Can you work these out from the model? Positions are in its coordinate system, mm. Face numbers are marked on the shaded views. A direction names the side the tool comes from. Coordinates: 2 decimals unless noted, no trailing zeros. Write each loop counter-clockwise with the first axis right and the second up, starting at its lowest first coordinate (ties: lowest second). Pieces come first, ordered by that corner, then holes. Notation, with made-up numbers: (32, 38.25) - (37, 38.25) arc R19 cw to (37, 63.25) - close; hole circle Ø8 at (5, 73). An arc over 180 degrees is marked (long way). Use one line per item in the form item = value. Start each with the question number.
(1) If we section it at D-D on z = 15.5: Please give me the cut outline in (x, y).
(2) Thinking about a two-plate mould opening in X: for the marked faces 4, 5 and 6, which applies, pulls with the +X half, pulls with the -X half, needs draft (parallel to the pull), parting line crosses it, or undercut?
(3) If we section it at B-B on x = 0: Please give me the cut outline in (y, z).
(4) On a 3-axis mill with a long thin cutter (end or side, diameter ignored), from which of +Z, -Z, +X, -X, +Y, -Y can I reach the whole of each face in a straight line? I mean the marked faces 1, 2 and 3. Say none if no direction works.
(5) If we section it at A-A on z = 2.5: Please give me the cut outline in (x, y).
(6) For pin 1 Ø6 at (x, z) = (19, -10) entering from +Y; pin 2 Ø12.5 at (x, y) = (3.5, -23) entering from +Z; pin 3 Ø6.5 at (y, z) = (-56.5, -4) entering from +X; pin 4 Ø10 at (x, y) = (2, -56) entering from +Z, each with a flat end and sliding along its axis, tell me the tip position at first contact or that it passes through.
(7) If I drill on probe 1 along Y at (x, z) = (0, 14.5); probe 2 along Y at (x, z) = (-0.5, 8); probe 3 along X at (y, z) = (-26, 9.5), over which ranges is the centre line in solid material (lowest first)? Write a range as from..to.
(8) If we section it at C-C on y = -20.5: Please give me the cut outline in (x, z).
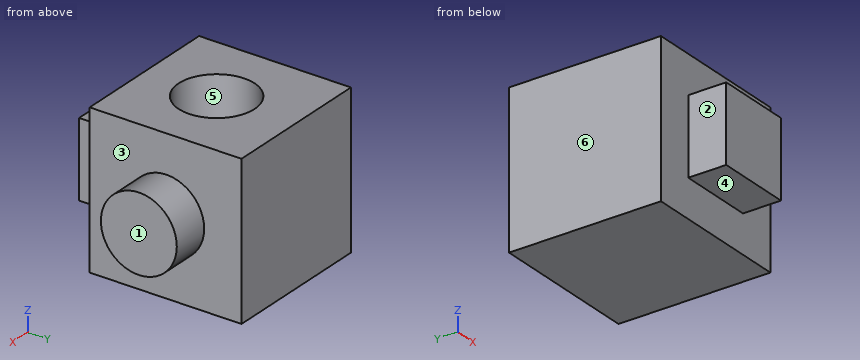
```python
from build123d import *

# Parameters (mm, degrees)
F0_W     = 50.8
F0_H     = 50.8
F1_DEPTH = 50.8
F2_W     = 25.4
F2_H     = 25.4
F3_DEPTH = 12.7
F4_R     = 12.7
F5_DEPTH = 12.7
F6_R     = 12.7
F7_DEPTH = 25.4


with BuildPart() as f1:
    # F0 (on Front) → F1 (new body)
    with BuildSketch(Plane.XZ):
        Rectangle(F0_W, F0_H)
    extrude(amount=F1_DEPTH)

    # F2 (on face) → F3 (join)
    with BuildSketch(Plane.XZ.offset(50.8)):
        Rectangle(F2_W, F2_H)
    extrude(amount=F3_DEPTH)

    # F4 (on face) → F5 (join)
    with BuildSketch(Plane.YZ.offset(25.4)):
        with Locations((-25.19346, 0)):
            Circle(F4_R)
    extrude(amount=F5_DEPTH)

    # F6 (on face) → F7 (cut)
    with BuildSketch(Plane.XY.offset(25.4)):
        with Locations((0, -26.625345)):
            Circle(F6_R)
    extrude(amount=-F7_DEPTH, mode=Mode.SUBTRACT)


solid = f1.part
```
Reported:
q1.outline = (-25.4, -50.8) - (25.4, -50.8) - (25.4, 0) - (-25.4, 0) - close; hole circle Ø25.4 at (0, -26.63)
q2.face_4 = needs draft
q2.face_5 = undercut
q2.face_6 = pulls with the -X half
q3.outline = (-63.5, -12.7) - (-50.8, -12.7) - (-50.8, -25.4) - (0, -25.4) - (0, 25.4) - (-13.93, 25.4) - (-13.93, 0) - (-39.33, 0) - (-39.33, 25.4) - (-50.8, 25.4) - (-50.8, 12.7) - (-63.5, 12.7) - close
q4.face_1 = +Z, -Z, +X, +Y, -Y
q4.face_2 = +Z, -Z, -X, -Y
q4.face_3 = +X
q5.outline = (-25.4, -50.8) - (-12.7, -50.8) - (-12.7, -63.5) - (12.7, -63.5) - (12.7, -50.8) - (25.4, -50.8) - (25.4, -37.64) - (38.1, -37.64) - (38.1, -12.74) - (25.4, -12.74) - (25.4, 0) - (-25.4, 0) - close; hole circle Ø25.4 at (0, -26.63)
q6.pin_1 = 0
q6.pin_2 = 0
q6.pin_3 = 12.7
q6.pin_4 = 12.7
q7.probe_1 = -50.8..-39.33, -13.93..0
q7.probe_2 = -63.5..-39.32, -13.94..0
q7.probe_3 = -25.4..-12.68, 12.68..38.1
q8.outline = (-25.4, -25.4) - (25.4, -25.4) - (25.4, -11.8) - (38.1, -11.8) - (38.1, 11.8) - (25.4, 11.8) - (25.4, 25.4) - (11.13, 25.4) - (11.13, 0) - (-11.13, 0) - (-11.13, 25.4) - (-25.4, 25.4) - close
